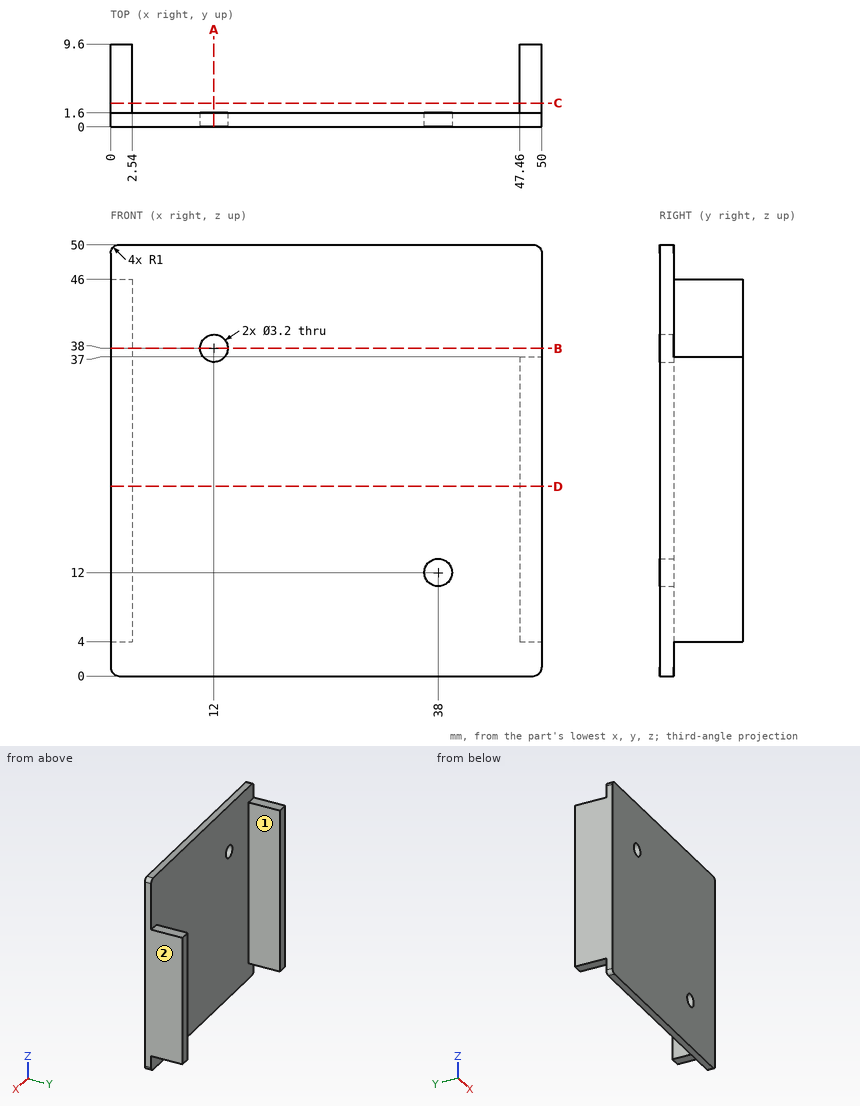
Job drawing, mm, ordinate dimensions from the low corner. One solid piece. A direction names the side the tool comes from. Round coordinates to 2 decimals unless told otherwise and drop trailing zeros. Loops run counter-clockwise (first coordinate to the right, second up) from the corner with the lowest first, then second, coordinate; pieces in that order, holes last. Notation, with made-up numbers: (-11.5, 40.25) -> (10.5, 40.25) arc R23 cw to (10.5, 57.25) -> close; hole circle Ø4 at (-6, -21). An arc over 180 degrees is marked (long way). One line per item, written item: value. Start each with the question number.
Q1. Cut at A-A on x = 12. List the corners of the cut face in (y, z), plus the area to 3 significant figures.
Q2. 3-axis set-ups, long thin cutter, end or side, ignore diameter. For the marked faces 1 and 2: which of +Z, -Z, +X, -X, +Y, -Y reach the whole face in a straight line?
Q3. Probe line 1 along Z through (x, y) = (12, 0.9); line 2 along Z through (x, y) = (38, 1.15). List the from-to ranges inside material, lowest first.
Q4. Cut at D-D on z = 22. List the corners of the cut face in (x, y).
Q5. Cut at C-C on y = 2.75. List the corners of the cut face in (x, z).
Q6. Cut at B-B on z = 38. List the corners of the cut face in (x, y).
Q7. Drop flat-ended pins along their axis: pin 1 Ø3 at (x, y) = (2, 7.5) entering from -Z; pin 2 Ø2 at (x, y) = (1, 4.5) entering from +Z; pin 3 Ø1 at (x, z) = (10, 16.5) entering from +Y. Give the stop position or say it passes through.
Computed:
1. outline: (0, 0) -> (1.6, 0) -> (1.6, 36.4) -> (0, 36.4) -> close; (0, 39.6) -> (1.6, 39.6) -> (1.6, 50) -> (0, 50) -> close
1. area: 74.9 mm²
2. face 1: +Z, -Z, +Y
2. face 2: +Z, -Z, +X, +Y, -Y
3. line 1: 0 to 36.4, 39.6 to 50
3. line 2: 0 to 10.4, 13.6 to 50
4. outline: (0, 0) -> (50, 0) -> (50, 9.6) -> (47.46, 9.6) -> (47.46, 1.6) -> (2.54, 1.6) -> (2.54, 9.6) -> (0, 9.6) -> close
5. outline: (0, 4) -> (2.54, 4) -> (2.54, 46) -> (0, 46) -> close; (47.46, 4) -> (50, 4) -> (50, 37) -> (47.46, 37) -> close
6. outline: (0, 0) -> (10.4, 0) -> (10.4, 1.6) -> (2.54, 1.6) -> (2.54, 9.6) -> (0, 9.6) -> close; (13.6, 0) -> (50, 0) -> (50, 1.6) -> (13.6, 1.6) -> close
7. pin 1: z = 4
7. pin 2: z = 46
7. pin 3: y = 1.6
